```python
from build123d import *

# Parameters (mm, degrees)
SKETCH_1_W = 4.5
SKETCH_1_H = 7


with BuildPart() as part:
    # 草图1 → 旋转3 (revolve)
    with BuildSketch(Plane.XY):
        with BuildLine():
            Line((7.5, 5), (7.5, -5))
            Line((7.5, -5), (13.75, -5))
            ThreePointArc((13.75, -5), (14.633883476, -4.633883476), (15, -3.75))
            Line((15, -3.75), (15, 3.75))
            ThreePointArc((15, 3.75), (14.633883476, 4.633883476), (13.75, 5))
            Line((13.75, 5), (7.5, 5))
        make_face()
        with Locations((11.25, 0)):
            Rectangle(SKETCH_1_W, SKETCH_1_H, mode=Mode.SUBTRACT)
    revolve(axis=Axis((0, -346.416551839, 0), (0, 1, 0)))


solid = part.part
```
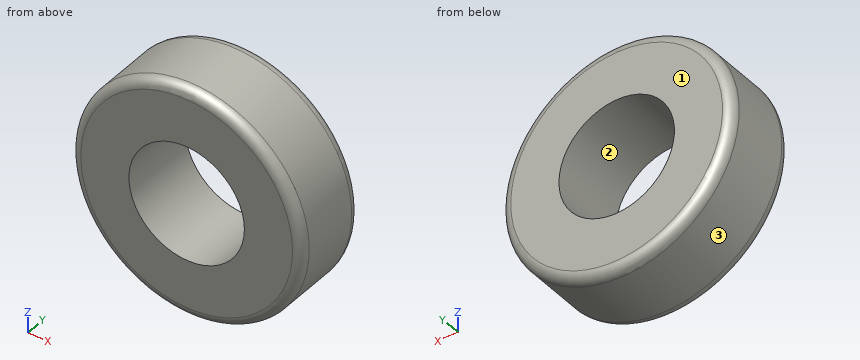
Geometry check sheet. Reference: the model listing, model coordinates, mm. Face numbers are marked on the shaded views. Coordinates: 2 decimals unless noted, no trailing zeros. Loops run counter-clockwise (first coordinate to the right, second up) from the corner with the lowest first, then second, coordinate; pieces in that order, holes last.
Item 1: Sectioned sample at A-A, the plane z = 0. Record the boundary of the cut face in (x, y).
Item 2: Release check for a two-part mould opening along Z. For the marked faces 1, 2 and 3 record: released by +Z, released by -Z, zero draft, split by the parting line, or undercut.
Item 3: Go/stop test with flat-tipped pins: pin 1 Ø1.5 at (y, z) = (0, 2) entering from -X; pin 2 Ø1.5 at (x, y) = (-11, 2) entering from -Z; pin 3 Ø1 at (y, z) = (-2, -2) entering from +X. Record where each tip stops, or that it passes through.
Item 4: Thickness scan on line 1 (X direction, y = 0.75, z = 0); line 2 (Y direction, x = -3.75, z = -12.5). Record the ranges inside material, lowest first.
Item 5: Sectioned sample at D-D, the plane z = 8. Count the separate pieces of the cut face and the enclosed holes in it, then the cut area to 3 significant figures.
Item 6: Sectioned sample at B-B, the plane x = 0. Record the boundary of the cut face in (y, z), then the cut area to 3 significant figures.
Item 7: Sectioned sample at C-C, the plane y = 1.25. Record the boundary of the cut face in (x, z).
Check result:
1. outline: (-15, -3.75) arc R1.25 ccw to (-13.75, -5) - (-7.5, -5) - (-7.5, 5) - (-13.75, 5) arc R1.25 ccw to (-15, 3.75) - close; (7.5, -5) - (13.75, -5) arc R1.25 ccw to (15, -3.75) - (15, 3.75) arc R1.25 ccw to (13.75, 5) - (7.5, 5) - close; hole (-13.5, -3.5) - (-9, -3.5) - (-9, 3.5) - (-13.5, 3.5) - close; hole (9, -3.5) - (13.5, -3.5) - (13.5, 3.5) - (9, 3.5) - close
2. face 1: zero draft
2. face 2: undercut
2. face 3: split by the parting line
3. pin 1: stops at x = -14.95
3. pin 2: stops at z = -10.95
3. pin 3: stops at x = 14.92
4. line 1: x = -15 to -13.5, -9 to -7.5, 7.5 to 9, 13.5 to 15
4. line 2: y = -5 to -3.5, 3.5 to 5
5. separate pieces: 1
5. enclosed holes: 2
5. area: 158 mm2
6. outline: (-5, -13.75) arc R1.25 ccw to (-3.75, -15) - (3.75, -15) arc R1.25 ccw to (5, -13.75) - (5, -7.5) - (-5, -7.5) - close; (-5, 7.5) - (5, 7.5) - (5, 13.75) arc R1.25 ccw to (3.75, 15) - (-3.75, 15) arc R1.25 ccw to (-5, 13.75) - close; hole (-3.5, -13.5) - (3.5, -13.5) - (3.5, -9) - (-3.5, -9) - close; hole (-3.5, 9) - (3.5, 9) - (3.5, 13.5) - (-3.5, 13.5) - close
6. area: 85.7 mm2
7. outline: circle Ø30 at (0, 0); circle Ø18 at (0, 0); hole circle Ø27 at (0, 0); hole circle Ø15 at (0, 0)
